The model under review builds one solid part; all positions refer to its coordinate system, in mm. Face numbers are marked on the shaded views. A direction names the side the tool comes from. Round coordinates to 2 decimals unless told otherwise and drop trailing zeros. Loops run counter-clockwise (first coordinate to the right, second up) from the corner with the lowest first, then second, coordinate; pieces in that order, holes last. Notation, with made-up numbers: (-30.75, -2.5) - (8.25, -2.5) arc R35 ccw to (8.25, 36.5) - close; hole circle Ø8 at (-21, 81.25). An arc over 180 degrees is marked (long way). Answer as CSV lines item,"result".
from build123d import *

# Parameters (mm, degrees)
F0_R     = 40
F1_DEPTH = 25


with BuildPart() as f1:
    # F0 (on Front) → F1 (new body)
    with BuildSketch(Plane.XZ):
        Circle(F0_R)
        with BuildLine():
            Line((24.370239, 27.5), (14.672255, -27.5))
            Line((14.672255, -27.5), (-9.697984, -27.5))
            Line((-9.697984, -27.5), (-2.185622, 15.104723))
            ThreePointArc((-2.185622, 15.104723), (2.94468, 23.990667), (12.586494, 27.5))
            Line((12.586494, 27.5), (24.370239, 27.5))
        make_face(mode=Mode.SUBTRACT)
    extrude(amount=F1_DEPTH)


solid = f1.part
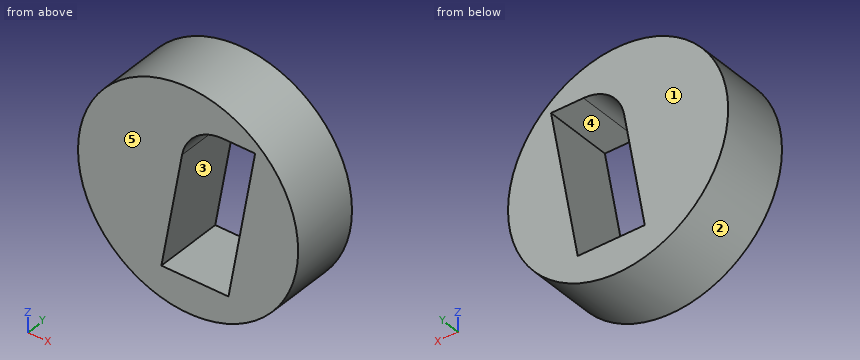
1. Wall thickness on probe 1 along X at (y, z) = (-1.25, 21); probe 2 along X at (y, z) = (-6, 25.5); probe 3 along Z at (x, y) = (9.5, -1.75): over which ranges is each line inside the solid? List them lowest first.
Numbers:
probe 1,"x = -34.04 to 0.23, 23.22 to 34.04"
probe 2,"x = -30.82 to 5.1, 24.02 to 30.82"
probe 3,"z = -38.86 to -27.5, 27.18 to 38.86"
2. Take a section at C-C (y = -13.5). State the section outline as (x, z) points, plus the area to 3 significant figures.
Numbers:
outline,"circle Ø80 at (0, 0); hole (-9.7, -27.5) - (14.67, -27.5) - (24.37, 27.5) - (12.59, 27.5) arc R15 ccw to (-2.19, 15.1) - close"
area,"3,720 mm²"
3. Clearance check with flat-ended pins moving along their axes: pin 1 (13 mm diameter, centred on x = 20.5, y = -16, fed in from -Z); pin 2 (12 mm diameter, centred on x = -23, y = -22, fed in from -Z); pin 3 (6 mm diameter, centred on x = 31.5, y = -13, fed in from +Z). State where each tip first meets the part, or that it passes through.
Numbers:
pin 1,"stops at z = -37.47"
pin 2,"stops at z = -36.21"
pin 3,"stops at z = 28.07"
4. Take a section at D-D (x = -14.5). State the section outline as (y, z) points.
Numbers:
outline,"(-25, -37.28) - (0, -37.28) - (0, 37.28) - (-25, 37.28) - close"
5. Tool access review of the marked faces 4 and 5: name each direction out of +Z, -Z, +X, -X, +Y, -Y from which nothing blocks a thin tool from reaching the whole face with its end or side.
Numbers:
face 4,"+Y, -Y"
face 5,"+Z, -Z, +X, -X, -Y"
6. Take a section at B-B (x = 0). State the section outline as (y, z) points.
Numbers:
outline,"(-25, -40) - (0, -40) - (0, -27.5) - (-25, -27.5) - close; (-25, 20.66) - (0, 20.66) - (0, 40) - (-25, 40) - close"
7. Take a section at A-A (z = 13). State the section outline as (x, y) points, plus the area to 3 significant figures.
Numbers:
outline,"(-37.83, -25) - (-2.56, -25) - (-2.56, 0) - (-37.83, 0) - close; (21.81, -25) - (37.83, -25) - (37.83, 0) - (21.81, 0) - close"
area,"1,280 mm²"
8. Draft analysis for pull direction Z (two halves, no side actions). For the marked faces 1, 2 and 3, state which applies: +Z half, -Z half, draft (parallel to the pull), parting line (faces both ways), or undercut.
Numbers:
face 1,"draft"
face 2,"parting line"
face 3,"undercut"
